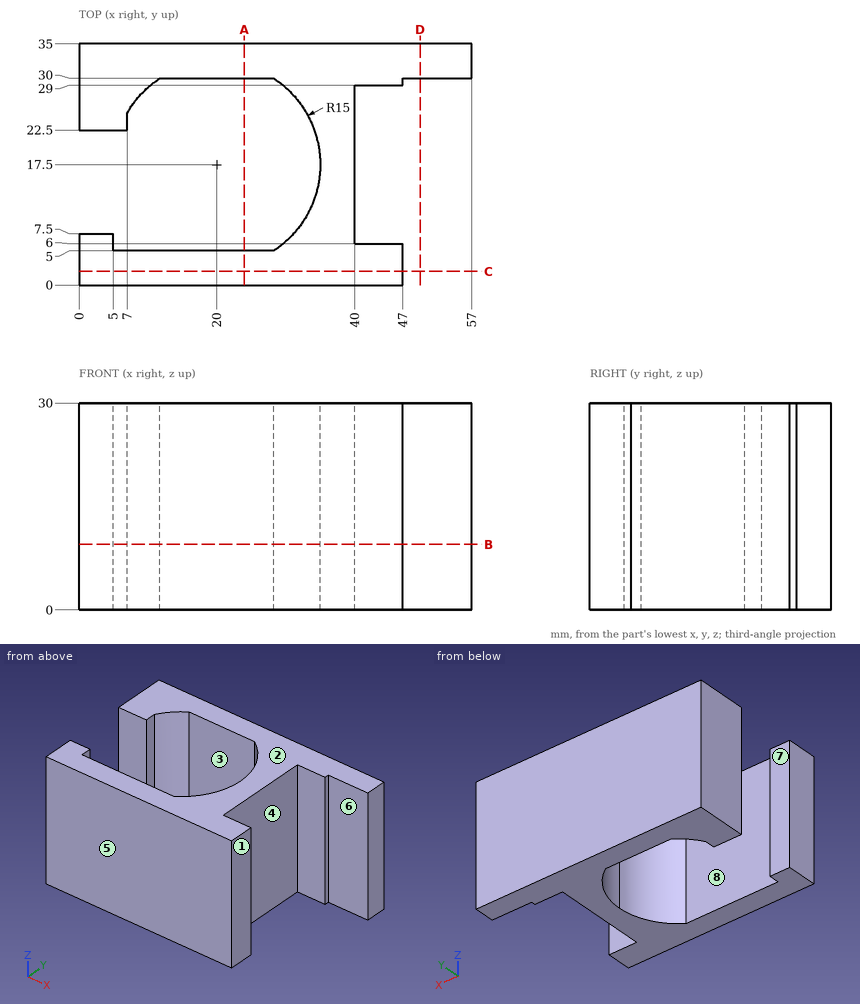
Could you check a few things on this drawing? It's one solid part, dimensions in mm from its lowest x, y, z. A direction names the side the tool comes from. Give positions to 0.01 mm unless a question says otherwise; leave off trailing zeros. Order: outer loops, then holes, each group sorted by start corner. A loop starts at its lowest first (then second) coordinate and runs counter-clockwise, first axis right, second up. Notation, with made-up numbers: (3, 75) - (35, 75) arc R16 cw to (35, 81) - close; hole circle Ø5 at (25.5, -3.75). An arc over 180 degrees is marked (long way). One line per item, written item: value. Start each with the question number.
1. Thinking about a two-plate mould opening in X: for the marked faces 1, 2 and 3, which applies, +X half, -X half, draft (parallel to the pull), parting line (faces both ways), or undercut?
2. If I drill on probe 1 along Y at (x, z) = (28, 7.5); probe 2 along Y at (x, z) = (47.5, 23.75); probe 3 along X at (y, z) = (26, 3.25), over which ranges is the centre line in solid material (lowest first)?
3. For P1, Ø0.5, axis at y = 29.5, z = 12, coming from the +X side; P2, Ø11.5, axis at y = 18.5, z = 14, coming from the +X side, each with a flat end and sliding along its axis, tell me the tip position at first contact or that it passes through.
4. Imagine slicing it at B-B on z = 9.5. List the corners of the cut face in (x, y) for me.
5. Imagine slicing it at A-A on x = 24. List the corners of the cut face in (y, z) for me.
6. Imagine slicing it at C-C on y = 2. List the corners of the cut face in (x, z) for me.
7. For the marked faces 4, 5, 6, 7 and 8, which set-ups out of +Z, -Z, +X, -X, +Y, -Y let a thin tool reach every point of the face, with its end or its side?
8. Imagine slicing it at D-D on x = 49.5. List the corners of the cut face in (y, z) for me, plus the area to 3 significant figures.
Values:
1. face 1: +X half
1. face 2: draft
1. face 3: undercut
2. probe 1: 0 to 5, 30 to 35
2. probe 2: 30 to 35
2. probe 3: 0 to 7.64, 32.36 to 40
3. P1: x = 47
3. P2: x = 40
4. outline: (0, 0) - (47, 0) - (47, 6) - (40, 6) - (40, 29) - (47, 29) - (47, 30) - (57, 30) - (57, 35) - (0, 35) - (0, 22.5) - (7, 22.5) - (7, 24.98) arc R15 cw to (11.71, 30) - (28.29, 30) arc R15 cw to (28.29, 5) - (5, 5) - (5, 7.5) - (0, 7.5) - close
5. outline: (0, 0) - (5, 0) - (5, 30) - (0, 30) - close; (30, 0) - (35, 0) - (35, 30) - (30, 30) - close
6. outline: (0, 0) - (47, 0) - (47, 30) - (0, 30) - close
7. face 4: +Z, -Z, +X
7. face 5: +Z, -Z, +X, -X, -Y
7. face 6: +Z, -Z, +X, -Y
7. face 7: +Z, -Z, -X
7. face 8: +Z, -Z
8. outline: (30, 0) - (35, 0) - (35, 30) - (30, 30) - close
8. area: 150 mm²
